Model file for the job. Use its own axes, mm. Round coordinates to 2 decimals unless told otherwise and drop trailing zeros. Put each result on its own line as item: value. Start each with the question number.
Q1. Probe L1, parallel to Z at x = 70, y = 0.75; L2, parallel to Z at x = 66.5, y = 5; L3, parallel to X at y = 4, z = -68.5. List the from-to ranges inside material, lowest first.
Q2. Flat gauge pins, fed straight in: P1, Ø1.5, axis at x = 111.5, y = 5, coming from the -Z side; P2, Ø2, axis at x = 127, y = 1.5, coming from the +Z side. Where does each tip first touch, or does it go through?
Q3. Cut at A-A, the plane x = 67. State how many separate pieces and enclosed holes the cut face has, and give its area (3 significant figures).
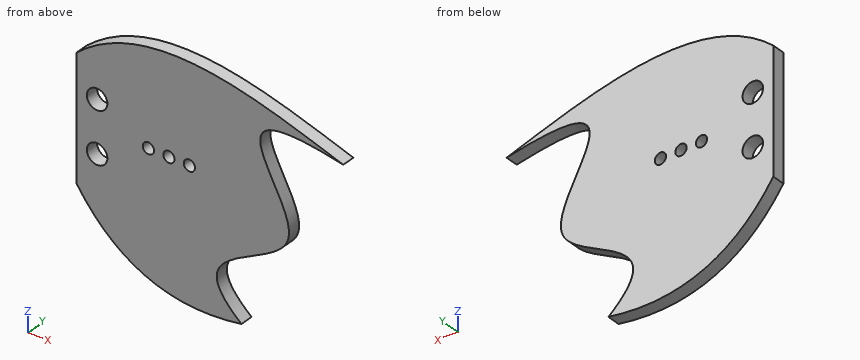
from build123d import *

# Parameters (mm, degrees)
BOSS_EXTRUDE1_DEPTH = 6.35
SKETCH3_R           = 2.75
CUT_EXTRUDE1_DEPTH  = 6.35
SKETCH4_R           = 5
CUT_EXTRUDE2_DEPTH  = 6.35
SKETCH5_R           = 2.75
CUT_EXTRUDE3_DEPTH  = 6.35


with BuildPart() as part:
    # Sketch2 → Boss-Extrude1 (new body)
    with BuildSketch(Plane(origin=(0, 0, 0), x_dir=(1, 0, 0), z_dir=(0, 1, 0))):
        with BuildLine():
            Line((56.391825432, 108.15139225), (56.391825432, 48.15139225))
            add(Edge.make_bspline(
                [(56.391825432, 48.15139225), (92.653221865, 15.965688803), (146.224111167, 35.551280798), (186.391825432, 48.15139225)],
                knots=[0, 0, 0, 0, 1, 1, 1, 1], degree=3))
            add(Edge.make_bspline(
                [(186.391825432, 48.15139225), (110.317005066, 33.459687001), (213.908429008, 108.517638804), (101.791603924, 111.907716317), (136.76058899, 140.645969256)],
                knots=[0, 0, 0, 0, 0.539021374, 1, 1, 1, 1], degree=3))
            add(Edge.make_bspline(
                [(56.391825432, 108.15139225), (85.056395763, 150.553247728), (136.76058899, 140.645969256)],
                knots=[0, 0, 0, 1, 1, 1], degree=2))
        make_face()
    extrude(amount=BOSS_EXTRUDE1_DEPTH)

    # Sketch3 → Cut-Extrude1 (cut)
    with BuildSketch(Plane(origin=(0, 0, 0), x_dir=(1, 0, 0), z_dir=(0, 1, 0))):
        with Locations((101.391825432, 78.15139225)):
            Circle(SKETCH3_R)
    extrude(amount=CUT_EXTRUDE1_DEPTH, mode=Mode.SUBTRACT)

    # Sketch4 → Cut-Extrude2 (cut)
    with BuildSketch(Plane(origin=(0, 0, 0), x_dir=(1, 0, 0), z_dir=(0, 1, 0))):
        with Locations((66.391825432, 90.65139225)):
            Circle(SKETCH4_R)
        with Locations((66.391825432, 65.65139225)):
            Circle(SKETCH4_R)
    extrude(amount=CUT_EXTRUDE2_DEPTH, mode=Mode.SUBTRACT)

    # Sketch5 → Cut-Extrude3 (cut)
    with BuildSketch(Plane(origin=(0, 0, 0), x_dir=(1, 0, 0), z_dir=(0, 1, 0))):
        with Locations((101.391825432, 78.15139225)):
            Circle(SKETCH5_R)
        with Locations((111.391825432, 78.15139225)):
            Circle(SKETCH5_R)
        with Locations((91.391825432, 78.15139225)):
            Circle(SKETCH5_R)
    extrude(amount=CUT_EXTRUDE3_DEPTH, mode=Mode.SUBTRACT)


solid = part.part
Ans:
1. L1: z = -124.17 to -94.11, -87.19 to -69.11, -62.19 to -38.77
1. L2: z = -120.74 to -95.65, -85.65 to -70.65, -60.65 to -40.72
1. L3: x = 56.39 to 62.28, 70.5 to 151.79
2. P1: stops at z = -142.32
2. P2: stops at z = -32.13
3. separate pieces: 3
3. enclosed holes: 0
3. area: 387 mm^2
